from build123d import *

# Parameters (mm, degrees)
SKETCH1_R           = 27
BOSS_EXTRUDE1_DEPTH = 2
BOSS_EXTRUDE2_START = 12.41
SKETCH2_R           = 27
SKETCH2_R_2         = 25
BOSS_EXTRUDE2_DEPTH = 12.41
BOSS_EXTRUDE3_START = -9
BOSS_EXTRUDE3_DEPTH = 9
CHAMFER1_SIZE       = 0.4


with BuildPart() as part:
    # Sketch1 → Boss-Extrude1 (new body)
    with BuildSketch(Plane.XY):
        Circle(SKETCH1_R)
        with BuildLine():
            Line((-9.232106781, -7.817893219), (-7.817893219, -9.232106781))
            ThreePointArc((-7.817893219, -9.232106781), (-7.49346987, -9.448879533), (-7.110786438, -9.525))
            Line((-7.110786438, -9.525), (7.110786438, -9.525))
            ThreePointArc((7.110786438, -9.525), (7.49346987, -9.448879533), (7.817893219, -9.232106781))
            Line((7.817893219, -9.232106781), (9.232106781, -7.817893219))
            ThreePointArc((9.232106781, -7.817893219), (9.448879533, -7.49346987), (9.525, -7.110786438))
            Line((9.525, -7.110786438), (9.525, 7.110786438))
            ThreePointArc((9.525, 7.110786438), (9.448879533, 7.49346987), (9.232106781, 7.817893219))
            Line((9.232106781, 7.817893219), (7.817893219, 9.232106781))
            ThreePointArc((7.817893219, 9.232106781), (7.49346987, 9.448879533), (7.110786438, 9.525))
            Line((7.110786438, 9.525), (-7.110786438, 9.525))
            ThreePointArc((-7.110786438, 9.525), (-7.49346987, 9.448879533), (-7.817893219, 9.232106781))
            Line((-7.817893219, 9.232106781), (-9.232106781, 7.817893219))
            ThreePointArc((-9.232106781, 7.817893219), (-9.448879533, 7.49346987), (-9.525, 7.110786438))
            Line((-9.525, 7.110786438), (-9.525, -7.110786438))
            ThreePointArc((-9.525, -7.110786438), (-9.448879533, -7.49346987), (-9.232106781, -7.817893219))
        make_face(mode=Mode.SUBTRACT)
    extrude(amount=BOSS_EXTRUDE1_DEPTH)

    # Sketch2 → Boss-Extrude2 (add)
    with BuildSketch(Plane(origin=(0, 0, 0), x_dir=(-1, 0, 0), z_dir=(0, 0, -1)).offset(BOSS_EXTRUDE2_START)):
        Circle(SKETCH2_R)
        with Locations(Location((0, 0, 0), (0, 0, 180))):
            Circle(SKETCH2_R_2, mode=Mode.SUBTRACT)
    extrude(amount=-BOSS_EXTRUDE2_DEPTH)

    # Sketch3 → Boss-Extrude3 (add)
    with BuildSketch(Plane.XY.offset(2).offset(BOSS_EXTRUDE3_START)):
        with BuildLine():
            Line((-7.110786438, -9.525), (7.110786438, -9.525))
            ThreePointArc((7.110786438, -9.525), (7.49346987, -9.448879533), (7.817893219, -9.232106781))
            Line((7.817893219, -9.232106781), (9.232106781, -7.817893219))
            ThreePointArc((9.232106781, -7.817893219), (9.448879533, -7.49346987), (9.525, -7.110786438))
            Line((9.525, -7.110786438), (9.525, 7.110786438))
            ThreePointArc((9.525, 7.110786438), (9.448879533, 7.49346987), (9.232106781, 7.817893219))
            Line((9.232106781, 7.817893219), (7.817893219, 9.232106781))
            ThreePointArc((7.817893219, 9.232106781), (7.49346987, 9.448879533), (7.110786438, 9.525))
            Line((7.110786438, 9.525), (-7.110786438, 9.525))
            ThreePointArc((-7.110786438, 9.525), (-7.49346987, 9.448879533), (-7.817893219, 9.232106781))
            Line((-7.817893219, 9.232106781), (-9.232106781, 7.817893219))
            ThreePointArc((-9.232106781, 7.817893219), (-9.448879533, 7.49346987), (-9.525, 7.110786438))
            Line((-9.525, 7.110786438), (-9.525, -7.110786438))
            ThreePointArc((-9.525, -7.110786438), (-9.448879533, -7.49346987), (-9.232106781, -7.817893219))
            Line((-9.232106781, -7.817893219), (-7.817893219, -9.232106781))
            ThreePointArc((-7.817893219, -9.232106781), (-7.49346987, -9.448879533), (-7.110786438, -9.525))
        make_face()
        Polygon((-7.069365081, -8.425), (7.069365081, -8.425), (8.425, -7.069365081), (8.425, 7.069365081), (7.069365081, 8.425), (-7.069365081, 8.425), (-8.425, 7.069365081), (-8.425, -7.069365081), align=None, mode=Mode.SUBTRACT)
    extrude(amount=BOSS_EXTRUDE3_DEPTH)

    # Chamfer1
    chamfer1_edges = [part.edges().sort_by_distance(p)[0] for p in [
        (-27, 0, 2),
        (-25, 0, 0),
        (27, 0, -12.41),
        (0, -9.525, -7),
        (7.49346987, -9.448879533, -7),
        (8.525, -8.525, -7),
        (9.448879533, -7.49346987, -7),
        (9.525, 0, -7),
        (9.448879533, 7.49346987, -7),
        (8.525, 8.525, -7),
        (7.49346987, 9.448879533, -7),
        (0, 9.525, -7),
        (-7.49346987, 9.448879533, -7),
        (-8.525, 8.525, -7),
        (-9.448879533, 7.49346987, -7),
        (-8.525, -8.525, -7),
        (-9.525, 0, -7),
        (-7.49346987, -9.448879533, -7),
        (-9.448879533, -7.49346987, -7),
        (-7.747182541, -7.747182541, 2),
        (-8.425, 0, 2),
        (-7.747182541, 7.747182541, 2),
        (0, 8.425, 2),
        (7.747182541, 7.747182541, 2),
        (8.425, 0, 2),
        (7.747182541, -7.747182541, 2),
        (0, -8.425, 2),
    ]]
    chamfer(chamfer1_edges, length=CHAMFER1_SIZE)


solid = part.part
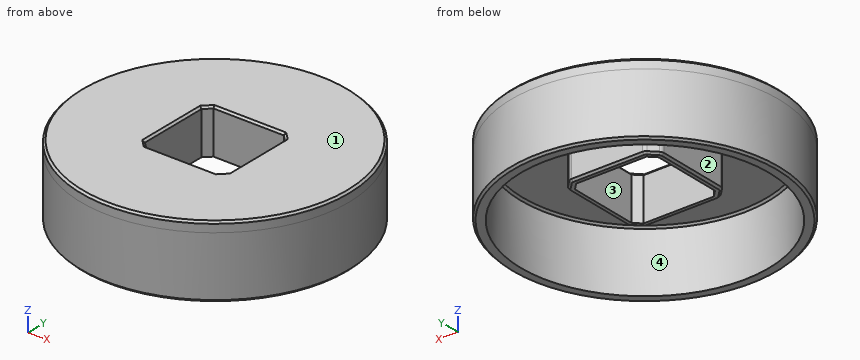
Design review of the part built by this model. Coordinates are the model's own, in mm. Face numbers are marked on the shaded views. A direction names the side the tool comes from. Coordinates: 2 decimals unless noted, no trailing zeros. Order: outer loops, then holes, each group sorted by start corner. A loop starts at its lowest first (then second) coordinate and runs counter-clockwise, first axis right, second up. Notation, with made-up numbers: M -11,28.25 L 19,28.25 A18 cw 19,45.25 Z; hole C 49.5,36 d3. An arc over 180 degrees is marked long. Use a Markdown table: item, result.
(1) Add section A-A (z = -1.25). Give the boundary of the cut face in (x, y) (3 decimals), then the cut area to 3 significant figures.
Worked answers:
| item | result |
|---|---|
| outline | C 0,0 d54; M -9.525,-7.111 A1 ccw -9.232,-7.818 L -7.818,-9.232 A1 ccw -7.111,-9.525 L 7.111,-9.525 A1 ccw 7.818,-9.232 L 9.232,-7.818 A1 ccw 9.525,-7.111 L 9.525,7.111 A1 ccw 9.232,7.818 L 7.818,9.232 A1 ccw 7.111,9.525 L -7.111,9.525 A1 ccw -7.818,9.232 L -9.232,7.818 A1 ccw -9.525,7.111 Z; hole C 0,0 d50; hole M -8.425,-7.069 L -7.069,-8.425 L 7.069,-8.425 L 8.425,-7.069 L 8.425,7.069 L 7.069,8.425 L -7.069,8.425 L -8.425,7.069 Z |
| area | 401 mm2 |
(2) For the marked faces 3 and 4, list the 3-axis set-ups (+Z, -Z, +X, -X, +Y, -Y) from which the entire face can be reached by the end or side of a thin tool; tool diameter is ignored.
Worked answers:
| item | result |
|---|---|
| face 3 | +Z, -Z |
| face 4 | -Z |
(3) Draft analysis for pull direction Y (two halves, no side actions). For the marked faces 1 and 2, state which applies: released by +Y, released by -Y, zero draft, split by the parting line, or undercut.
Worked answers:
| item | result |
|---|---|
| face 1 | zero draft |
| face 2 | undercut |
(4) Add section B-B (x = 0). Give the boundary of the cut face in (y, z) (3 decimals), then the cut area to 3 significant figures.
Worked answers:
| item | result |
|---|---|
| outline | M -27,-12.01 L -26.6,-12.41 L -25,-12.41 L -25,-0.4 L -24.6,0 L -9.525,0 L -9.525,-6.6 L -9.125,-7 L -8.425,-7 L -8.425,1.6 L -8.825,2 L -26.6,2 L -27,1.6 Z; M 8.425,-7 L 9.125,-7 L 9.525,-6.6 L 9.525,0 L 24.6,0 L 25,-0.4 L 25,-12.41 L 26.6,-12.41 L 27,-12.01 L 27,1.6 L 26.6,2 L 8.825,2 L 8.425,1.6 Z |
| area | 139 mm2 |
(5) For P1, Ø2, axis at x = -15, y = -3, coming from the -Z side; P2, Ø6, axis at x = -5.5, z = -6.5, coming from the -Y side; P3, Ø5.5, axis at x = -3, z = -2, coming from the -Y side; P4, Ø9, axis at x = 0, y = 0, coming from the -Z side, all flat-tipped, find the tip position at first contact; note any pin that passes through.
Worked answers:
| item | result |
|---|---|
| P1 | stops at z = 0 |
| P2 | stops at y = -26.88 |
| P3 | stops at y = -27 |
| P4 | passes through |
(6) Wall thickness on probe 1 along Y at (x, z) = (0, -4.25) (3 decimals); probe 2 along Y at (x, z) = (0, -7.5); probe 3 along X at (y, z) = (14, -6.5): over which ranges is each line inside the solid? List them lowest first.
Worked answers:
| item | result |
|---|---|
| probe 1 | y = -27 to -25, -9.525 to -8.425, 8.425 to 9.525, 25 to 27 |
| probe 2 | y = -27 to -25, 25 to 27 |
| probe 3 | x = -23.09 to -20.71, 20.71 to 23.09 |
(7) Add section D-D (z = -10.75). Give the boundary of the cut face in (x, y), then the cut area to 3 significant figures.
Worked answers:
| item | result |
|---|---|
| outline | C 0,0 d54; hole C 0,0 d50 |
| area | 327 mm2 |
